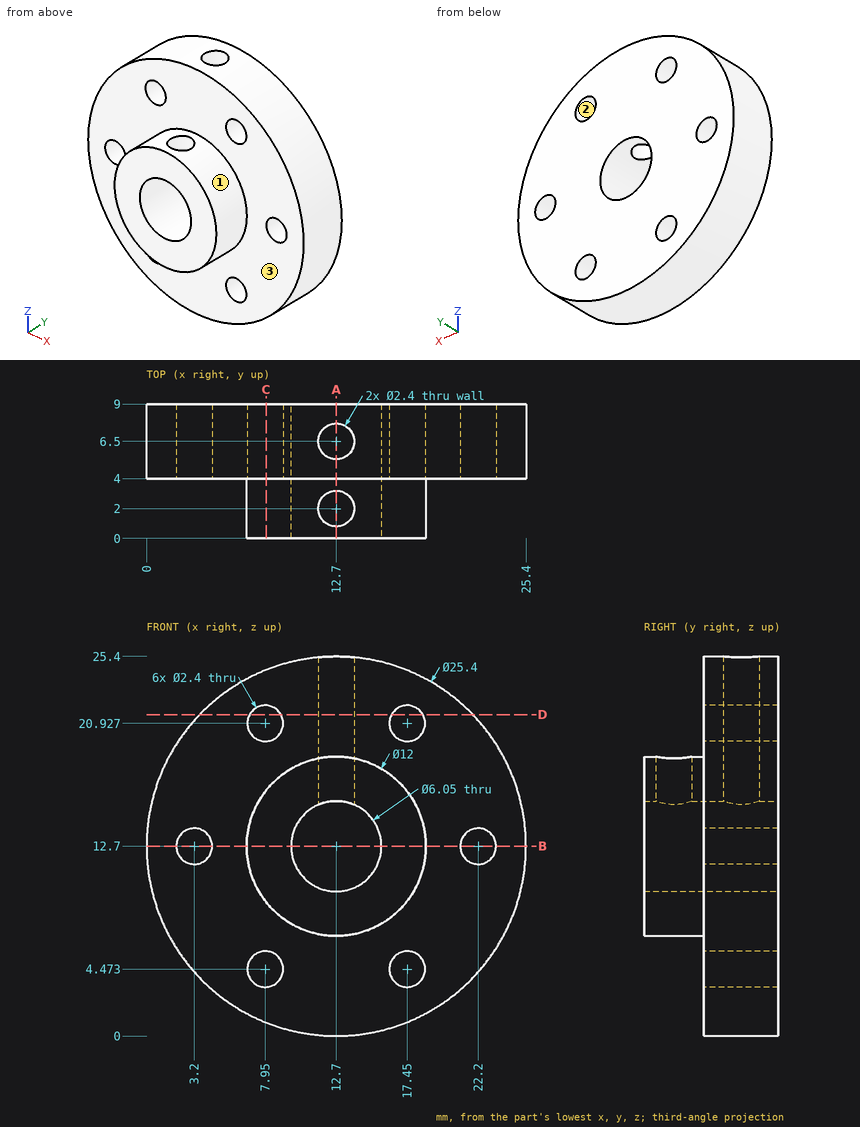
Geometry: see drawing. Coordinates: mm, zero at the bounding-box minimum. Coordinates: 2 decimals unless noted, no trailing zeros. Order: outer loops, then holes, each group sorted by start corner. A loop starts at its lowest first (then second) coordinate and runs counter-clockwise, first axis right, second up. Notation, with made-up numbers: M 82.25,7 L 121.25,7 A26 ccw 121.25,41 Z; hole C 48,68.25 d4. An arc over 180 degrees is marked long. Write each question's results on one line, items separated by ' | '. Start each with the question number.
1) Draft query along X for the marked faces 1, 2 and 3. Return one class per face: released by +X, released by -X, zero draft, split by the parting line, or undercut.
2) Section query A-A (x = 12.7). Return the cut outline in (y, z) (3 decimals).
3) Section query D-D (z = 21.5). Return the cut outline in (x, y).
4) Line query: line 1 (Y direction, x = 12.7, z = 16.85); line 2 (Y direction, x = 12.7, z = 21.75); line 3 (Z direction, x = 17.45, y = 7.45). Output: solid intervals per line, ascending. Write a range as from..to.
5) Contact query for flat-ended pins moving along their axis: pin 1 Ø2 at (x, y) = (17, 5.5) entering from +Z; pin 2 Ø2 at (x, z) = (3.2, 12.7) entering from +Y; pin 3 Ø2 at (y, z) = (8, 11) entering from +X; pin 4 Ø3 at (x, z) = (17.45, 4.47) entering from -Y. Output: stop coordinate, or through.
6) Section query C-C (x = 8). Return the cut outline in (y, z), plus the area to 3 significant figures.
7) Section query B-B (z = 12.7). Return the cut outline in (x, y) (3 decimals).
Answers:
1) face 1: split by the parting line | face 2: undercut | face 3: zero draft
2) outline: M 0,6.7 L 4,6.7 L 4,0 L 9,0 L 9,9.675 L 0,9.675 Z; M 0,15.725 L 0.8,15.725 L 0.8,18.7 L 0,18.7 Z; M 3.2,15.725 L 5.3,15.725 L 5.3,25.4 L 4,25.4 L 4,18.7 L 3.2,18.7 Z; M 7.7,15.725 L 9,15.725 L 9,25.4 L 7.7,25.4 Z
3) outline: M 3.54,4 L 6.9,4 L 6.9,9 L 3.54,9 Z; M 9,4 L 16.4,4 L 16.4,9 L 9,9 Z; M 18.5,4 L 21.86,4 L 21.86,9 L 18.5,9 Z; hole C 12.7,6.5 d2.4
4) line 1: y = 0..0.8, 3.2..5.3, 7.7..9 | line 2: y = 4..5.3, 7.7..9 | line 3: z = 0.92..3.27, 5.67..19.73, 22.13..24.48
5) pin 1: stops at z = 24.96 | pin 2: passes through | pin 3: stops at x = 25.38 | pin 4: stops at y = 4
6) outline: M 0,8.97 L 4,8.97 L 4,5.67 L 9,5.67 L 9,19.73 L 4,19.73 L 4,16.43 L 0,16.43 Z; M 4,0.9 L 9,0.9 L 9,3.27 L 4,3.27 Z; M 4,22.13 L 9,22.13 L 9,24.5 L 4,24.5 Z | area: 124 mm^2
7) outline: M 0,4 L 2,4 L 2,9 L 0,9 Z; M 4.4,4 L 6.7,4 L 6.7,0 L 9.675,0 L 9.675,9 L 4.4,9 Z; M 15.725,0 L 18.7,0 L 18.7,4 L 21,4 L 21,9 L 15.725,9 Z; M 23.4,4 L 25.4,4 L 25.4,9 L 23.4,9 Z
